Check sheet for the modelled part. Datum: model origin and axes. Units: mm. Face numbers are marked on the shaded views. A direction names the side the tool comes from. Round coordinates to 2 decimals unless told otherwise and drop trailing zeros. Order: outer loops, then holes, each group sorted by start corner. A loop starts at its lowest first (then second) coordinate and runs counter-clockwise, first axis right, second up. Notation, with made-up numbers: (84, 10) -> (138, 10) arc R21 ccw to (138, 31) -> close; hole circle Ø10 at (49.5, 2.5). An arc over 180 degrees is marked (long way). Answer in a Markdown table with one row per item.
```python
from build123d import *

# Parameters (mm, degrees)
OBJ1       = 12
SKETCH_03_SCREW_SHAFT_PROFILE_R  = 3.8
PAD_04_SCREW_SHAFT_DEPTH         = 38
SKETCH_05_PRESSURE_PAD_PROFILE_R = 12
PAD_06_PRESSURE_PAD_DEPTH        = 4


with BuildPart() as part:
    with BuildSketch(Plane.XY):
        Polygon((24, 0), (20.32462, 2.675787), (23.18222, 6.211657), (18.93953, 7.84501), (20.78461, 12), (16.263743, 12.479609), (16.970563, 16.970563), (12.479609, 16.263743), (12, 20.78461), (7.84501, 18.93953), (6.211657, 23.18222), (2.675787, 20.32462), (0, 24), (-2.675787, 20.32462), (-6.211657, 23.18222), (-7.84501, 18.93953), (-12, 20.78461), (-12.479609, 16.263743), (-16.970563, 16.970563), (-16.263743, 12.479609), (-20.78461, 12), (-18.93953, 7.84501), (-23.18222, 6.211657), (-20.32462, 2.675787), (-24, 0), (-20.32462, -2.675787), (-23.18222, -6.211657), (-18.93953, -7.84501), (-20.78461, -12), (-16.263743, -12.479609), (-16.970563, -16.970563), (-12.479609, -16.263743), (-12, -20.78461), (-7.84501, -18.93953), (-6.211657, -23.18222), (-2.675787, -20.32462), (0, -24), (2.675787, -20.32462), (6.211657, -23.18222), (7.84501, -18.93953), (12, -20.78461), (12.479609, -16.263743), (16.970563, -16.970563), (16.263743, -12.479609), (20.78461, -12), (18.93953, -7.84501), (23.18222, -6.211657), (20.32462, -2.675787), align=None)
    extrude(amount=OBJ1)

    # Sketch_03_Screw_Shaft_Profile → Pad_04_Screw_Shaft (join)
    with BuildSketch(Plane.XY.offset(12)):
        Circle(SKETCH_03_SCREW_SHAFT_PROFILE_R)
    extrude(amount=PAD_04_SCREW_SHAFT_DEPTH)

    # Sketch_05_Pressure_Pad_Profile → Pad_06_Pressure_Pad (join)
    with BuildSketch(Plane.XY.offset(50)):
        Circle(SKETCH_05_PRESSURE_PAD_PROFILE_R)
    extrude(amount=PAD_06_PRESSURE_PAD_DEPTH)


solid = part.part
```
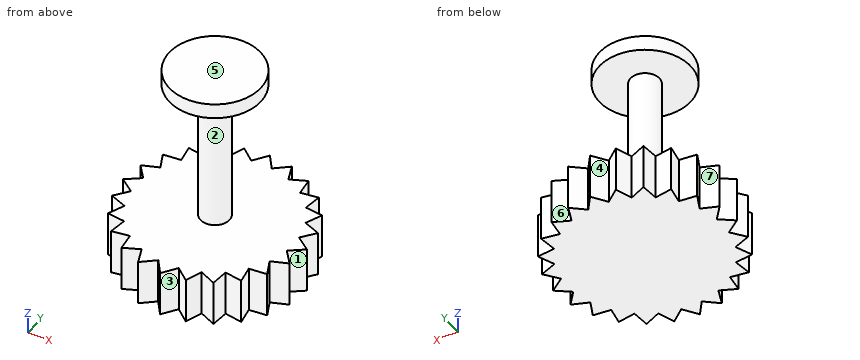
(1) Section check B-B on y = 10.5. Record the boundary of the cut face in (x, z), plus the area to 3 significant figures.
Solutions:
| item | result |
|---|---|
| outline | (-20.12, 0) -> (20.12, 0) -> (20.12, 12) -> (-20.12, 12) -> close; (-5.81, 50) -> (5.81, 50) -> (5.81, 54) -> (-5.81, 54) -> close |
| area | 529 mm^2 |
(2) Section check D-D on y = -15. Record the boundary of the cut face in (x, z).
Solutions:
| item | result |
|---|---|
| outline | (-16.66, 0) -> (16.66, 0) -> (16.66, 12) -> (-16.66, 12) -> close |
(3) Scan lines: probe 1 along Z at (x, y) = (7, 9.5); probe 2 along Z at (x, y) = (-19.5, -1); probe 3 along Y at (x, z) = (-3.5, 14). Record each from-to range of solid material in increasing order. Write a range as from..to.
Solutions:
| item | result |
|---|---|
| probe 1 | 0..12, 50..54 |
| probe 2 | 0..12 |
| probe 3 | -1.48..1.48 |
(4) Draft check along Y on the marked faces 5, 6 and 7. Enter one of: pulls with the +Y half, pulls with the -Y half, needs draft (parallel to the pull), parting line crosses it, or undercut.
Solutions:
| item | result |
|---|---|
| face 5 | needs draft |
| face 6 | pulls with the +Y half |
| face 7 | undercut |
(5) Section check C-C on z = 15. Record the boundary of the cut face in (x, y).
Solutions:
| item | result |
|---|---|
| outline | circle Ø7.6 at (0, 0) |
(6) Section check A-A on x = -10. Record the boundary of the cut face in (y, z).
Solutions:
| item | result |
|---|---|
| outline | (-19.9, 0) -> (19.9, 0) -> (19.9, 12) -> (-19.9, 12) -> close; (-6.63, 50) -> (6.63, 50) -> (6.63, 54) -> (-6.63, 54) -> close |
(7) Depth check by flat-ended pin: pin 1 Ø4 at (x, z) = (2.5, 40) entering from -Y; pin 2 Ø5 at (x, y) = (4.5, 15.5) entering from +Z; pin 3 Ø10 at (y, z) = (-10, 13.5) entering from -X. Enter the tip coordinate at first touch or a pass-through.
Solutions:
| item | result |
|---|---|
| pin 1 | y = -3.77 |
| pin 2 | z = 12 |
| pin 3 | x = -23.18 |
(8) Tool access check on the marked faces 1, 2, 3 and 4. Record the directions out of +Z, -Z, +X, -X, +Y, -Y that give a thin tool (end or side, any length) a straight path to the whole face; none if there is none.
Solutions:
| item | result |
|---|---|
| face 1 | +Z, -Z, +X |
| face 2 | none |
| face 3 | +Z, -Z, -Y |
| face 4 | +Z, -Z, +Y |
